Geometry: final body of the model. Coordinates: model frame, mm. A direction names the side the tool comes from. Coordinates: 2 decimals unless noted, no trailing zeros. Write each loop counter-clockwise with the first axis right and the second up, starting at its lowest first coordinate (ties: lowest second). Pieces come first, ordered by that corner, then holes. Notation, with made-up numbers: (83.25, 54) - (130.25, 54) arc R7 ccw to (130.25, 65) - close; hole circle Ø7 at (-7, 17). An arc over 180 degrees is marked (long way). Answer as a JSON object with one key per item and string values. Group by question number.
Item 1: Line query: line 1 along Y through (x, z) = (135.85, 3.3); line 2 along Y through (x, z) = (127.5, 30); line 3 along Y through (x, z) = (196.9, 242.5). Output: solid intervals per line, ascending. Write a range as from..to.
Item 2: Set-up query: faces 1 (the flat face through (200, 2, 148)), 2 (the flat face through (-195, -2, 150)), 3 (the cylindrical face through (197.54, -128.57, 244.13)). Return all of +Z, -Z, +X, -X, +Y, -Y with unobstructed straight access to the full face (end or side cutting, diameter ignored); none if empty.
Item 3: Section A-A on y = -121.25. Return loops of the section in (x, z).
Item 4: Mould query, pull axis Y, two halves, no side actions, for faces 4 (the flat face through (195, 2, 150)), 5 (the flat face through (3, -150, 148)), 6 (the flat face through (-200, -2, 148)), 7 (the flat face through (-3, 150, 148)). Classes: pulls with the +Y half, pulls with the -Y half, needs draft (parallel to the pull), parting line crosses it, or undercut.
Item 5: Section D-D on x = 77.5. Return loops of the section in (y, z), and give its area (3 significant figures).
Item 6: Section C-C on y = -61. Return loops of the section in (x, z), and give its area (3 significant figures).
Item 7: First-contact query: pin 1 Ø7 at (x, y) = (135.85, 85.85) entering from +Z. Flat tip, straight axial feed; report the tip coordinate or a pass-through.
Item 8: Section B-B on z = 57.5. Return loops of the section in (x, y).
Autodesk Inventor part; units mm, degrees
ref_plane "YZ Plane" through (0, 0, 0) normal (1, 0, 0) x (0, 1, 0)
ref_plane "XZ Plane" through (0, 0, 0) normal (0, 1, 0) x (-1, 0, 0)
ref_plane "XY Plane" through (0, 0, 0) normal (0, 0, 1) x (1, 0, 0)
sketch "Sketch2" plane through (0, 0, 0) normal (0, 0, 1) x (1, 0, 0)
  line L0 (200, -150) -> (-200, -150)
  line L1 (-200, -150) -> (-200, 150)
  line L2 (-200, 150) -> (200, 150)
  line L3 (200, 150) -> (200, -150)
  line L4 (200, -150) -> (-200, 150) construction
  line L5 (-200, -150) -> (200, 150) construction
  point P0 (0, 0)
  dimension "d0" = 400
  dimension "d1" = 300
extrude "Base" add sketch "Sketch2" along normal blind 300
shell "Shell1" thickness 5 removed faces 1 at (66.6667, -50, 300)
sketch "Sketch3" plane through (0, 0, 0) normal (0, 0, -1) x (-1, 0, 0)
  circle A0 centre (-167.85, 85.85) radius 2.15
  line L0 (-200, 150) -> (200, 150) construction
  line L1 (-200, 150) -> (200, 150) construction
  line L2 (200, 150) -> (200, -150) construction
  line L3 (200, -150) -> (-200, -150) construction
  line L4 (-200, -150) -> (-200, 150) construction
  circle A1 centre (-135.85, 85.85) radius 2.15
  circle A2 centre (-167.85, 117.85) radius 2.15
  circle A3 centre (-135.85, 117.85) radius 2.15
  point P0 (0, 0)
  dimension "d5" = 4.3
  dimension "d8" = 32
  dimension "d11" = 32
  dimension "d14" = 32.15
  dimension "d15" = 32.15
extrude "40 mm fan mout holes" cut sketch "Sketch3" against normal up to surface (5 mm away)
sketch "Sketch4" plane through (200, -150, 0) normal (1, 0, 0) x (0, 0, -1)
  circle A0 centre (-242.5, 28.75) radius 7.5
  line L0 (-300, 0) -> (-300, 300)
  line L1 (0, 0) -> (-300, 0)
  circle A1 centre (-222.5, 28.75) radius 7.5
  point P0 (0, 150)
  dimension "d18" = 15
  dimension "d19" = 57.5
  dimension "d20" = 28.75
  dimension "d23" = 20
extrude "Cable Holes" cut sketch "Sketch4" against normal up to surface (5 mm away)
equation "\"d15\" = d14"
equation "\"d20\" = 0.5 * d19"
properties part number "mouse_SP_box"
Checks:
{
 "1": {"line 1": "-150..83.7, 88..115.7, 120..150", "line 2": "-150..-145, 145..150", "line 3": "-150..-128.75, -113.75..150"},
 "2": {"face 1": "+Z, -Z, +X, +Y, -Y", "face 2": "+Z", "face 3": "+X"},
 "3": {"outline": "(-200, 0) - (200, 0) - (200, 215) - (195, 215) - (195, 5) - (-195, 5) - (-195, 300) - (-200, 300) - close; (195, 230) - (200, 230) - (200, 235) - (195, 235) - close; (195, 250) - (200, 250) - (200, 300) - (195, 300) - close"},
 "4": {"face 4": "undercut", "face 5": "pulls with the -Y half", "face 6": "needs draft", "face 7": "pulls with the +Y half"},
 "5": {"outline": "(-150, 0) - (150, 0) - (150, 300) - (145, 300) - (145, 5) - (-145, 5) - (-145, 300) - (-150, 300) - close", "area": "4,450 mm^2"},
 "6": {"outline": "(-200, 0) - (200, 0) - (200, 300) - (195, 300) - (195, 5) - (-195, 5) - (-195, 300) - (-200, 300) - close", "area": "4,950 mm^2"},
 "7": {"pin 1": "z = 5"},
 "8": {"outline": "(-200, -150) - (200, -150) - (200, 150) - (-200, 150) - close; hole (-195, -145) - (195, -145) - (195, 145) - (-195, 145) - close"}
}
